from build123d import *

# Parameters (mm, degrees)
BOSS_EXTRUDE1_DEPTH = 50
SKETCH2_W           = 21
SKETCH2_H           = 56
CUT_EXTRUDE1_DEPTH  = 14
CUT_EXTRUDE2_DEPTH  = 40
CUT_EXTRUDE3_START  = -45
CUT_EXTRUDE3_DEPTH  = 45
SKETCH5_R           = 2
CUT_EXTRUDE4_DEPTH  = 10
SKETCH6_R           = 2
CUT_EXTRUDE5_DEPTH  = 5


with BuildPart() as part:
    # Sketch1 → Boss-Extrude1 (new body)
    with BuildSketch(Plane.XY):
        with BuildLine():
            Line((-40, 50), (40, 50))
            ThreePointArc((40, 50), (47.071067812, 47.071067812), (50, 40))
            Line((50, 40), (50, -40))
            ThreePointArc((50, -40), (47.071067812, -47.071067812), (40, -50))
            Line((40, -50), (-40, -50))
            ThreePointArc((-40, -50), (-47.071067812, -47.071067812), (-50, -40))
            Line((-50, -40), (-50, 40))
            ThreePointArc((-50, 40), (-47.071067812, 47.071067812), (-40, 50))
        make_face()
    extrude(amount=BOSS_EXTRUDE1_DEPTH)

    # Sketch2 → Cut-Extrude1 (cut)
    with BuildSketch(Plane.XY.offset(50)):
        with Locations((0, -5)):
            Rectangle(SKETCH2_W, SKETCH2_H)
    extrude(amount=-CUT_EXTRUDE1_DEPTH, mode=Mode.SUBTRACT)

    # Sketch3 → Cut-Extrude2 (cut)
    with BuildSketch(Plane.XY.offset(36)):
        Polygon((-10.5, 16.220000255), (-10.5, -25.279999745), (10.5, -25.279999745), (10.5, 16.220000255), (2.75, 16.220000255), (2.728552587, 23.719969589), (-2.771447413, 23.719969589), (-2.75, 16.220000255), align=None)
    extrude(amount=-CUT_EXTRUDE2_DEPTH, mode=Mode.SUBTRACT)

    # Sketch4 → Cut-Extrude3 (cut)
    with BuildSketch(Plane.XY.offset(50).offset(CUT_EXTRUDE3_START)):
        with BuildLine():
            Line((40, -50), (25, -50))
            Line((25, -50), (25, 50))
            Line((25, 50), (40, 50))
            ThreePointArc((40, 50), (47.071067812, 47.071067812), (50, 40))
            Line((50, 40), (50, -40))
            ThreePointArc((50, -40), (47.071067812, -47.071067812), (40, -50))
        make_face()
        with BuildLine():
            Line((-40, -50), (-25, -50))
            Line((-25, -50), (-25, 50))
            Line((-25, 50), (-40, 50))
            ThreePointArc((-40, 50), (-47.071067812, 47.071067812), (-50, 40))
            Line((-50, 40), (-50, -40))
            ThreePointArc((-50, -40), (-47.071067812, -47.071067812), (-40, -50))
        make_face()
    extrude(amount=CUT_EXTRUDE3_DEPTH, mode=Mode.SUBTRACT)

    # Sketch5 → Cut-Extrude4 (cut)
    with BuildSketch(Plane.XY.offset(36)):
        with Locations((-5, 19.5)):
            Circle(SKETCH5_R)
        with Locations((5, 19.5)):
            Circle(SKETCH5_R)
        with Locations((-5, -29.3)):
            Circle(SKETCH5_R)
        with Locations((5, -29.3)):
            Circle(SKETCH5_R)
    extrude(amount=-CUT_EXTRUDE4_DEPTH, mode=Mode.SUBTRACT)

    # Sketch6 → Cut-Extrude5 (cut)
    with BuildSketch(Plane.XY.offset(5)):
        with Locations((-32.783708715, 43.482376607)):
            Circle(SKETCH6_R)
        with Locations((-32.783708715, -41.517623393)):
            Circle(SKETCH6_R)
        with Locations((32.216291285, -41.364915091)):
            Circle(SKETCH6_R)
        with Locations((32.216291285, 43.635084909)):
            Circle(SKETCH6_R)
    extrude(amount=-CUT_EXTRUDE5_DEPTH, mode=Mode.SUBTRACT)


solid = part.part
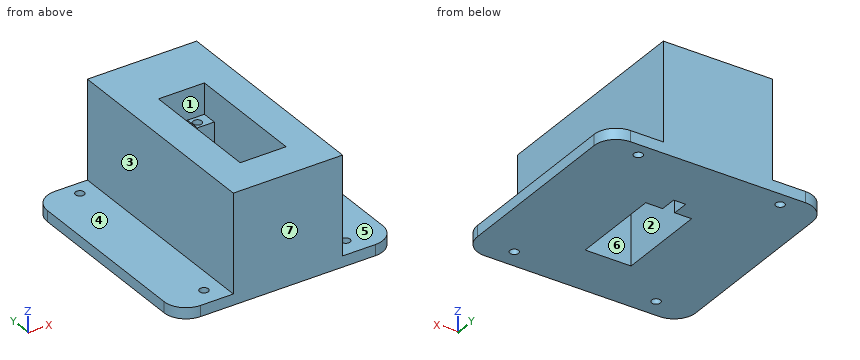
The model under review builds one solid part; all positions refer to its coordinate system, in mm. Face numbers are marked on the shaded views. A direction names the side the tool comes from. Round coordinates to 2 decimals unless told otherwise and drop trailing zeros. Loops run counter-clockwise (first coordinate to the right, second up) from the corner with the lowest first, then second, coordinate; pieces in that order, holes last. Notation, with made-up numbers: M 25.5,-1 L 75.5,-1 A18 cw 75.5,31 Z; hole C 28,41 d7. An arc over 180 degrees is marked long. Answer as CSV lines item,"result". Start each with the question number.
Item 1: Consider section A-A (x = -5). Write out the cut boundary in (y, z).
Item 2: Consider section B-B (z = 33). Write out the cut boundary in (x, y).
Item 3: Insertion check: P1, Ø8.5, axis at x = -3, y = -28, coming from the +Z side; P2, Ø1.2, axis at x = 6, y = -29, coming from the +Z side; P3, Ø4.5, axis at x = -32.78, y = 43.48, coming from the +Z side. Each pin has a flat end and moves straight along its axis. Give the tip position at first contact, or say it passes through.
Item 4: Consider section C-C (y = -29.3). Write out the cut boundary in (x, z), then the cut area to 3 significant figures.
Item 5: Mouldability with a two-part tool opening along X and no side actions: class the marked faces 1, 2, 3 and 4 as released by +X, released by -X, zero draft, split by the parting line, or undercut.
Item 6: Wall thickness on line 1 (Y direction, x = -5, z = 31.75); line 2 (X direction, y = -6, z = 19); line 3 (X direction, y = 19, z = 29): over which ranges is each line inside the solid? List them lowest first. Write a range as [from, to].
Item 7: For the marked faces 5, 6 and 7, list the 3-axis set-ups (+Z, -Z, +X, -X, +Y, -Y) from which the entire face can be reached by the end or side of a thin tool; tool diameter is ignored.
Item 8: Consider section D-D (y = 5.5). Write out the cut boundary in (x, z).
Answer:
1,outline,"M -50,0 L -25.28,0 L -25.28,36 L -27.3,36 L -27.3,26 L -31.3,26 L -31.3,36 L -33,36 L -33,50 L -50,50 Z; M 16.22,0 L 50,0 L 50,50 L 23,50 L 23,36 L 21.5,36 L 21.5,26 L 17.5,26 L 17.5,36 L 16.22,36 Z"
2,outline,"M -25,-50 L 25,-50 L 25,50 L -25,50 Z; hole M -10.5,-25.28 L 10.5,-25.28 L 10.5,16.22 L 2.75,16.22 L 2.73,23.72 L -2.77,23.72 L -2.75,16.22 L -10.5,16.22 Z; hole C -5,-29.3 d4; hole C -5,19.5 d4; hole C 5,-29.3 d4; hole C 5,19.5 d4"
3,P1,"stops at z = 36"
3,P2,"stops at z = 26"
3,P3,"stops at z = 5"
4,outline,"M -50,0 L 50,0 L 50,5 L 25,5 L 25,50 L 10.5,50 L 10.5,36 L 7,36 L 7,26 L 3,26 L 3,36 L -3,36 L -3,26 L -7,26 L -7,36 L -10.5,36 L -10.5,50 L -25,50 L -25,5 L -50,5 Z"
4,area,"2,380 mm^2"
5,face 1,"undercut"
5,face 2,"undercut"
5,face 3,"released by -X"
5,face 4,"zero draft"
6,line 1,"y = [-50, -31.3], [-27.3, -25.28], [16.22, 17.5], [21.5, 50]"
6,line 2,"x = [-25, -10.5], [10.5, 25]"
6,line 3,"x = [-25, -6.94], [-3.06, -2.76], [2.74, 3.06], [6.94, 25]"
7,face 5,"+Z, +X, +Y, -Y"
7,face 6,"+Z, -Z"
7,face 7,"+Z, -Z, +X, -X, -Y"
8,outline,"M -50,0 L -10.5,0 L -10.5,50 L -25,50 L -25,5 L -50,5 Z; M 10.5,0 L 50,0 L 50,5 L 25,5 L 25,50 L 10.5,50 Z"
